```python
from build123d import *

# Parameters (mm, degrees)
SKETCH_2_R          = 1.6
SKETCH_2_W          = 15
SKETCH_2_H          = 15
CUT_EXTRUDE_1_DEPTH = 29.049064156
HOLE_WIZARD_M3_1_D  = 2.5
SKETCH_6_R          = 1.5
CUT_EXTRUDE_2_DEPTH = 11
FILLET_1_R          = 1


with BuildPart() as part:
    # 草图1 → 旋转1 (revolve)
    with BuildSketch(Plane(origin=(0, 0, 0), x_dir=(0, 0, -1), z_dir=(1, 0, 0)), mode=Mode.PRIVATE) as revolve_1_sk:
        Polygon((0, 0), (15.5, 0), (15.5, 6.5), (12.5, 6.5), (12.5, 17.5), (0, 17.5), align=None)
    revolve(revolve_1_sk.sketch.rotate(Axis((0, 25.607258106, 0), (0, -1, 0)), 180), axis=Axis((0, 25.607258106, 0), (0, -1, 0)))

    # 草图2 → 切除-拉伸1 (cut, through all)
    with BuildSketch(Plane(origin=(0, 0, 0), x_dir=(1, 0, 0), z_dir=(0, 1, 0))):
        with Locations((6.36862915, 6.36862915)):
            Circle(SKETCH_2_R)
        with Locations((-6.36862915, 6.36862915)):
            Circle(SKETCH_2_R)
        with Locations((-6.36862915, -6.36862915)):
            Circle(SKETCH_2_R)
        with Locations((6.36862915, -6.36862915)):
            Circle(SKETCH_2_R)
        Rectangle(SKETCH_2_W, SKETCH_2_H)
    extrude(amount=CUT_EXTRUDE_1_DEPTH, mode=Mode.SUBTRACT)

    # M3 螺纹孔1 (through all)
    with Locations(Plane(origin=(0, 0, 0), x_dir=(-1, 0, 0), z_dir=(0, -1, 0))):
        with Locations((12, 0), (0, 12), (-12, 0), (0, -12)):
            Hole(HOLE_WIZARD_M3_1_D / 2)

    # 草图6 → 切除-拉伸2 (cut)
    with BuildSketch(Plane(origin=(0, 17.5, 0), x_dir=(1, 0, 0), z_dir=(0, 1, 0))):
        with Locations((-12, 0)):
            Circle(SKETCH_6_R)
        with Locations((0, 12)):
            Circle(SKETCH_6_R)
        with Locations((12, 0)):
            Circle(SKETCH_6_R)
        with Locations((0, -12)):
            Circle(SKETCH_6_R)
    extrude(amount=-CUT_EXTRUDE_2_DEPTH, mode=Mode.SUBTRACT)

    # 圆角1
    fillet_1_edges = [part.edges().sort_by_distance(p)[0] for p in [
        (-12.416666667, 12, 1.440968039),
        (-12.416666667, 12, -1.440968039),
        (-1.440968039, 12, -12.416666667),
        (1.440968039, 12, -12.416666667),
        (12.416666667, 12, -1.440968039),
        (12.416666667, 12, 1.440968039),
        (-1.440968039, 12, 12.416666667),
        (1.440968039, 12, 12.416666667),
    ]]
    fillet(fillet_1_edges, radius=FILLET_1_R)


solid = part.part
```
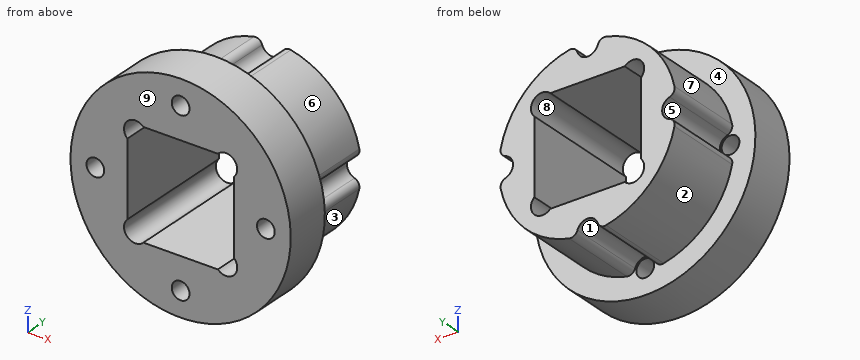
Geometry check sheet. Reference: the model listing, model coordinates, mm. Face numbers are marked on the shaded views. A direction names the side the tool comes from. Give positions to 0.01 mm unless a question says otherwise; leave off trailing zeros. Loops run counter-clockwise (first coordinate to the right, second up) from the corner with the lowest first, then second, coordinate; pieces in that order, holes last. Notation, with made-up numbers: M 7.5,11.5 L 66.5,11.5 A19 cw 66.5,47.5 Z; hole C 38.5,56.25 d9. An arc over 180 degrees is marked long. Answer as CSV lines item,"result".
Item 1: Depth check by flat-ended pin: P1, Ø1, axis at y = 12, z = -10, coming from the +X side; P2, Ø1.5, axis at x = -8.5, y = 4, coming from the +Z side; P3, Ø3, axis at y = 6, z = -11.5, coming from the +X side. Enter the tip coordinate at first touch or a pass-through.
Values:
P1,"stops at x = 8.12"
P2,"stops at z = 13.42"
P3,"stops at x = 11.84"
Item 2: Release check for a two-part mould opening along X. For the marked faces 6, 7, 8 and 9 record: pulls with the +X half, pulls with the -X half, needs draft (parallel to the pull), parting line crosses it, or undercut.
Values:
face 6,"pulls with the +X half"
face 7,"pulls with the -X half"
face 8,"undercut"
face 9,"needs draft"
Item 3: Cross-section at A-A on z = 0. Record the cut outline in (x, y), and give its area (4 significant figures).
Values:
outline,"M -15.5,0 L -13.25,0 L -13.25,6.5 L -15.5,6.5 Z; M -10.75,0 L -7.5,0 L -7.5,17.5 L -10.5,17.5 L -10.5,6.5 L -10.75,6.5 Z; M 7.5,0 L 10.75,0 L 10.75,6.5 L 10.5,6.5 L 10.5,17.5 L 7.5,17.5 Z; M 13.25,0 L 15.5,0 L 15.5,6.5 L 13.25,6.5 Z"
area,"137.5 mm²"
Item 4: Material ranges on line 1 (X direction, y = 13.5, z = -10); line 2 (Z direction, x = -1, y = 8.5); line 3 (Z direction, x = -12, y = 5), recorded low to high.
Values:
line 1,"x = -7.5 to 7.5"
line 2,"z = -10.88 to -7.5, 7.5 to 10.88"
line 3,"z = -9.81 to -1.25, 1.25 to 9.81"
Item 5: Cross-section at D-D on z = -6. Record the cut outline in (x, y).
Values:
outline,"M -14.29,0 L -7.93,0 L -7.93,17.5 L -10.97,17.5 L -10.97,6.5 L -14.29,6.5 Z; M 7.93,0 L 14.29,0 L 14.29,6.5 L 10.97,6.5 L 10.97,17.5 L 7.93,17.5 Z"
Item 6: Cross-section at C-C on y = 4. Record the cut outline in (x, z), and give its area (3 significant figures).
Values:
outline,"C 0,0 d31; hole C -12,0 d2.5; hole M -7.5,-5.24 A1.6 ccw -5.24,-7.5 L 5.24,-7.5 A1.6 ccw 7.5,-5.24 L 7.5,5.24 A1.6 ccw 5.24,7.5 L -5.24,7.5 A1.6 ccw -7.5,5.24 Z; hole C 0,-12 d2.5; hole C 0,12 d2.5; hole C 12,0 d2.5"
area,"504 mm²"
Item 7: Access from +Z, -Z, +X, -X, +Y, -Y to the whole of each face (thin tool, end or side, straight path). Record for the marked faces 1, 2, 3, 4 and 5.
Values:
face 1,"-Z, +Y"
face 2,"-Z, -X, +Y"
face 3,"-Z, +X, +Y"
face 4,"+Y"
face 5,"-X, +Y"
Item 8: Cross-section at B-B on x = 7. Record the cut outline in (y, z).
Values:
outline,"M 0,-13.83 L 6.5,-13.83 L 6.5,-10.36 L 17.5,-10.36 L 17.5,-7.84 L 0,-7.84 Z; M 0,7.84 L 17.5,7.84 L 17.5,10.36 L 6.5,10.36 L 6.5,13.83 L 0,13.83 Z"
